The model under review builds one solid part; all positions refer to its coordinate system, in mm. Round coordinates to 2 decimals unless told otherwise and drop trailing zeros. Loops run counter-clockwise (first coordinate to the right, second up) from the corner with the lowest first, then second, coordinate; pieces in that order, holes last. Notation, with made-up numbers: (81.25, 55.25) -> (126.25, 55.25) arc R20 cw to (126.25, 81.25) -> close; hole circle Ø10 at (36.25, -24.5). An arc over 180 degrees is marked (long way). Use a Markdown table: item, result. Add a question column.
1) Consider section C-C on x = -54. Give the boundary of the cut face in (y, z).
2) Insertion check: pin 1 (1.4 mm diameter, centred on x = -20, y = 1, fed in from +Z); pin 2 (1.4 mm diameter, centred on x = -34.5, y = 1, fed in from -Z); pin 3 (1.2 mm diameter, centred on y = 1, z = -5.5, fed in from +X). Each pin has a flat end and moves straight along its axis. Give the tip position at first contact, or say it passes through.
3) Consider section A-A on x = -34. Give the boundary of the cut face in (y, z).
4) Consider section B-B on z = -6.25. Give the boundary of the cut face in (x, y), plus the area to 3 significant figures.
5) Wall thickness on probe 1 along X at (y, z) = (0.35, -6.25); probe 2 along Z at (x, y) = (-50, 0.2); probe 3 along Z at (x, y) = (-89, 0.35): over which ranges is each line inside the solid? List them lowest first.
6) Consider section D-D on y = 2.2. State how many separate pieces and enclosed holes the cut face has, plus the area to 3 significant figures.
from build123d import *

# Parameters (mm, degrees)
BOSS_EXTRUDE1_DEPTH = 2.7


with BuildPart() as part:
    # Sketch1 → Boss-Extrude1 (new body)
    with BuildSketch(Plane(origin=(0, 0, 0), x_dir=(1, 0, 0), z_dir=(0, 1, 0))):
        Polygon((4, 2.833333333), (4, 12.366666667), (6.7, 12.366666667), (6.7, 21.9), (4, 21.9), (4, 19.2), (-36.5, 19.2), (-36.5, 21.9), (-77, 21.9), (-77, 19.2), (-117.5, 19.2), (-117.5, 12.366666667), (-117.5, 2.833333333), (-117.5, -4), (-77, -4), (-77, -6.7), (-36.5, -6.7), (-36.5, -4), (4, -4), (4, -6.7), (6.7, -6.7), (6.7, 2.833333333), align=None)
        with BuildLine():
            Line((-91.627899854, 8.1), (-85.172100146, 8.1))
            ThreePointArc((-85.172100146, 8.1), (-84.626142897, 7.873857103), (-84.4, 7.327899854))
            Line((-84.4, 7.327899854), (-84.4, 4.872100146))
            ThreePointArc((-84.4, 4.872100146), (-84.626142897, 4.326142897), (-85.172100146, 4.1))
            Line((-85.172100146, 4.1), (-91.627899854, 4.1))
            ThreePointArc((-91.627899854, 4.1), (-92.173857103, 4.326142897), (-92.4, 4.872100146))
            Line((-92.4, 4.872100146), (-92.4, 7.327899854))
            ThreePointArc((-92.4, 7.327899854), (-92.173857103, 7.873857103), (-91.627899854, 8.1))
        make_face(mode=Mode.SUBTRACT)
        with BuildLine():
            Line((-73.627899854, 8.1), (-67.172100146, 8.1))
            ThreePointArc((-67.172100146, 8.1), (-66.626142897, 7.873857103), (-66.4, 7.327899854))
            Line((-66.4, 7.327899854), (-66.4, 4.872100146))
            ThreePointArc((-66.4, 4.872100146), (-66.626142897, 4.326142897), (-67.172100146, 4.1))
            Line((-67.172100146, 4.1), (-73.627899854, 4.1))
            ThreePointArc((-73.627899854, 4.1), (-74.173857103, 4.326142897), (-74.4, 4.872100146))
            Line((-74.4, 4.872100146), (-74.4, 7.327899854))
            ThreePointArc((-74.4, 7.327899854), (-74.173857103, 7.873857103), (-73.627899854, 8.1))
        make_face(mode=Mode.SUBTRACT)
        with BuildLine():
            Line((-55.627899854, 8.1), (-49.172100146, 8.1))
            ThreePointArc((-49.172100146, 8.1), (-48.626142897, 7.873857103), (-48.4, 7.327899854))
            Line((-48.4, 7.327899854), (-48.4, 4.872100146))
            ThreePointArc((-48.4, 4.872100146), (-48.626142897, 4.326142897), (-49.172100146, 4.1))
            Line((-49.172100146, 4.1), (-55.627899854, 4.1))
            ThreePointArc((-55.627899854, 4.1), (-56.173857103, 4.326142897), (-56.4, 4.872100146))
            Line((-56.4, 4.872100146), (-56.4, 7.327899854))
            ThreePointArc((-56.4, 7.327899854), (-56.173857103, 7.873857103), (-55.627899854, 8.1))
        make_face(mode=Mode.SUBTRACT)
        with BuildLine():
            Line((-37.627899854, 8.1), (-31.172100146, 8.1))
            ThreePointArc((-31.172100146, 8.1), (-30.626142897, 7.873857103), (-30.4, 7.327899854))
            Line((-30.4, 7.327899854), (-30.4, 4.872100146))
            ThreePointArc((-30.4, 4.872100146), (-30.626142897, 4.326142897), (-31.172100146, 4.1))
            Line((-31.172100146, 4.1), (-37.627899854, 4.1))
            ThreePointArc((-37.627899854, 4.1), (-38.173857103, 4.326142897), (-38.4, 4.872100146))
            Line((-38.4, 4.872100146), (-38.4, 7.327899854))
            ThreePointArc((-38.4, 7.327899854), (-38.173857103, 7.873857103), (-37.627899854, 8.1))
        make_face(mode=Mode.SUBTRACT)
        with BuildLine():
            Line((-15.627899854, 8.1), (-9.172100146, 8.1))
            ThreePointArc((-9.172100146, 8.1), (-8.626142897, 7.873857103), (-8.4, 7.327899854))
            Line((-8.4, 7.327899854), (-8.4, 4.872100146))
            ThreePointArc((-8.4, 4.872100146), (-8.626142897, 4.326142897), (-9.172100146, 4.1))
            Line((-9.172100146, 4.1), (-15.627899854, 4.1))
            ThreePointArc((-15.627899854, 4.1), (-16.173857103, 4.326142897), (-16.4, 4.872100146))
            Line((-16.4, 4.872100146), (-16.4, 7.327899854))
            ThreePointArc((-16.4, 7.327899854), (-16.173857103, 7.873857103), (-15.627899854, 8.1))
        make_face(mode=Mode.SUBTRACT)
    extrude(amount=BOSS_EXTRUDE1_DEPTH)


solid = part.part
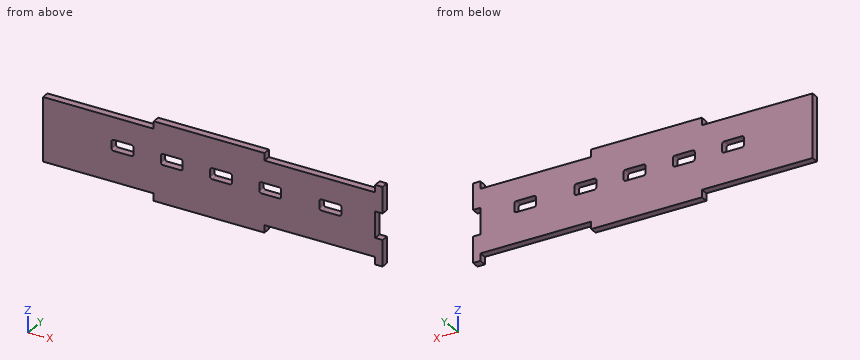
Result set:
| question | item | result |
|---|---|---|
| 1 | outline | (0, -21.9) -> (2.7, -21.9) -> (2.7, -8.1) -> (0, -8.1) -> close; (0, -4.1) -> (2.7, -4.1) -> (2.7, 6.7) -> (0, 6.7) -> close |
| 2 | pin 1 | z = 4 |
| 2 | pin 2 | z = -19.2 |
| 2 | pin 3 | x = 4 |
| 3 | outline | (0, -19.2) -> (2.7, -19.2) -> (2.7, -8.1) -> (0, -8.1) -> close; (0, -4.1) -> (2.7, -4.1) -> (2.7, 4) -> (0, 4) -> close |
| 4 | outline | (-117.5, 0) -> (-92.4, 0) -> (-92.4, 2.7) -> (-117.5, 2.7) -> close; (-84.4, 0) -> (-74.4, 0) -> (-74.4, 2.7) -> (-84.4, 2.7) -> close; (-66.4, 0) -> (-56.4, 0) -> (-56.4, 2.7) -> (-66.4, 2.7) -> close; (-48.4, 0) -> (-38.4, 0) -> (-38.4, 2.7) -> (-48.4, 2.7) -> close; (-30.4, 0) -> (-16.4, 0) -> (-16.4, 2.7) -> (-30.4, 2.7) -> close; (-8.4, 0) -> (4, 0) -> (4, 2.7) -> (-8.4, 2.7) -> close |
| 4 | area | 220 mm2 |
| 5 | probe 1 | -117.5 to -92.4, -84.4 to -74.4, -66.4 to -56.4, -48.4 to -38.4, -30.4 to -16.4, -8.4 to 4 |
| 5 | probe 2 | -21.9 to -8.1, -4.1 to 6.7 |
| 5 | probe 3 | -19.2 to -8.1, -4.1 to 4 |
| 6 | separate pieces | 1 |
| 6 | enclosed holes | 5 |
| 6 | area | 2,930 mm2 |
